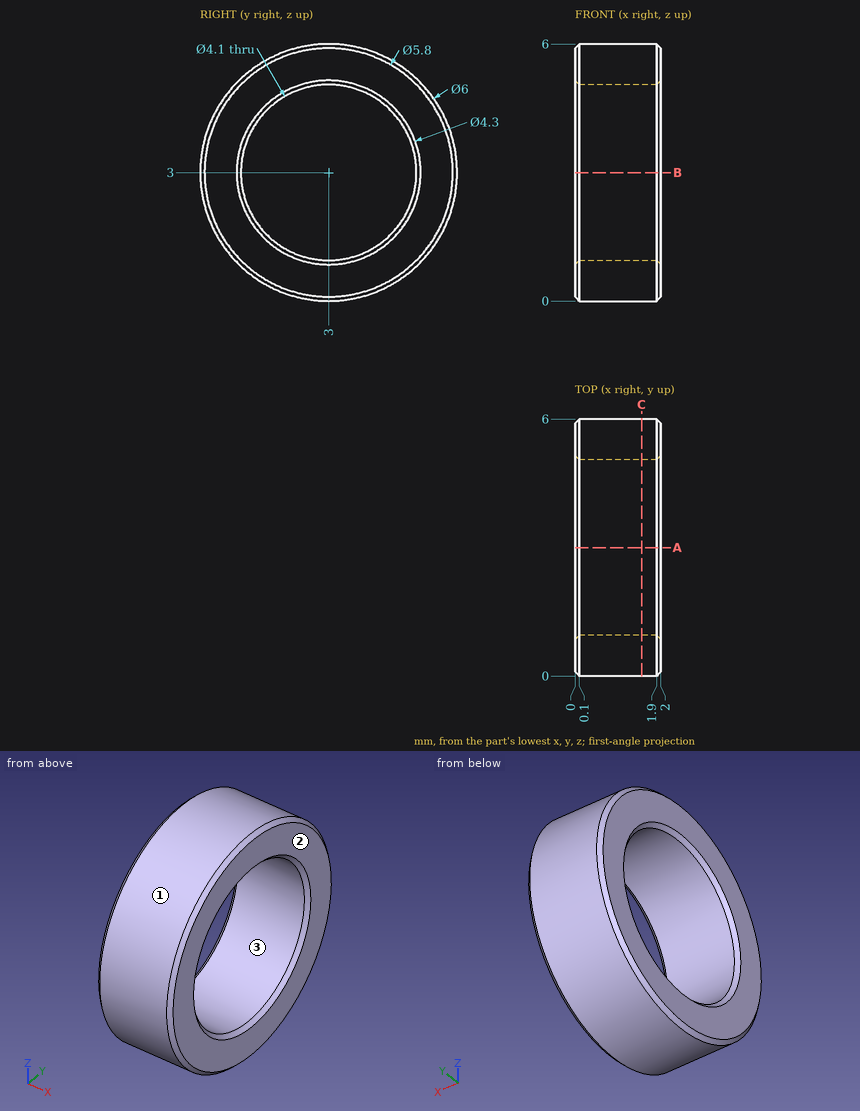
Could you check a few things on this drawing? It's one solid part, dimensions in mm from its lowest x, y, z. Round coordinates to 2 decimals unless told otherwise and drop trailing zeros. Order: outer loops, then holes, each group sorted by start corner. A loop starts at its lowest first (then second) coordinate and runs counter-clockwise, first axis right, second up.
(1) Please list where these lines run through material, in increasing order: line 1 along Y through (x, z) = (1.5, 3); line 2 along Z through (x, y) = (0.75, 2.45); line 3 along Y through (x, z) = (1.4, 4.2).
Response values:
line 1: y = 0 to 0.95, 5.05 to 6
line 2: z = 0.05 to 1.03, 4.97 to 5.95
line 3: y = 0.25 to 1.34, 4.66 to 5.75
(2) Imagine slicing it at C-C (x = 1.55). Write out the boundary of the cut face in (y, z).
Response values:
outline: circle Ø6 at (3, 3); hole circle Ø4.1 at (3, 3)
(3) If we mould it in two halves opening along Y, with no side actions, what happens to the marked faces 1, 2 and 3? For each: released by +Y, released by -Y, zero draft, split by the parting line, or undercut.
Response values:
face 1: split by the parting line
face 2: zero draft
face 3: undercut
(4) Imagine slicing it at A-A (y = 3). Write out the boundary of the cut face in (x, z).
Response values:
outline: (0, 0.1) - (0.1, 0) - (1.9, 0) - (2, 0.1) - (2, 0.85) - (1.9, 0.95) - (0.1, 0.95) - (0, 0.85) - close; (0, 5.15) - (0.1, 5.05) - (1.9, 5.05) - (2, 5.15) - (2, 5.9) - (1.9, 6) - (0.1, 6) - (0, 5.9) - close
(5) I'm going to push a flat-ended pin straight in: pin 1 (1 mm diameter, centred on x = 1.5, y = 4.5, fed in from -Z). Where does the tip first touch, or does it pass through?
Response values:
pin 1: stops at z = 0.17
